Drawing for the job (mm, zero at the part's lowest x, y, z). Give positions to 0.01 mm unless a question says otherwise; leave off trailing zeros. Loops run counter-clockwise (first coordinate to the right, second up) from the corner with the lowest first, then second, coordinate; pieces in that order, holes last. Notation, with made-up numbers: M 45,66.5 L 88,66.5 A10 cw 88,76.5 Z; hole C 53.25,1.5 d4. An arc over 180 degrees is marked long. Use CSV: the item, a comma, the result in double quotes. Start each with the question number.
(1) Slice it at A-A on y = 7.5. List the corners of the cut face in (x, z), and give its area (3 significant figures).
(2) Slice it at C-C on x = 10. List the corners of the cut face in (y, z).
(3) Slice it at B-B on z = 13. List the corners of the cut face in (x, y), and give its area (3 significant figures).
(4) Wall check: line 1 along X through (y, z) = (8, 56.5); line 2 along X through (y, z) = (3.5, 51); line 3 along Z through (x, y) = (14, 0.5). Give the ranges that are in metal, low to high. Write a range as from..to.
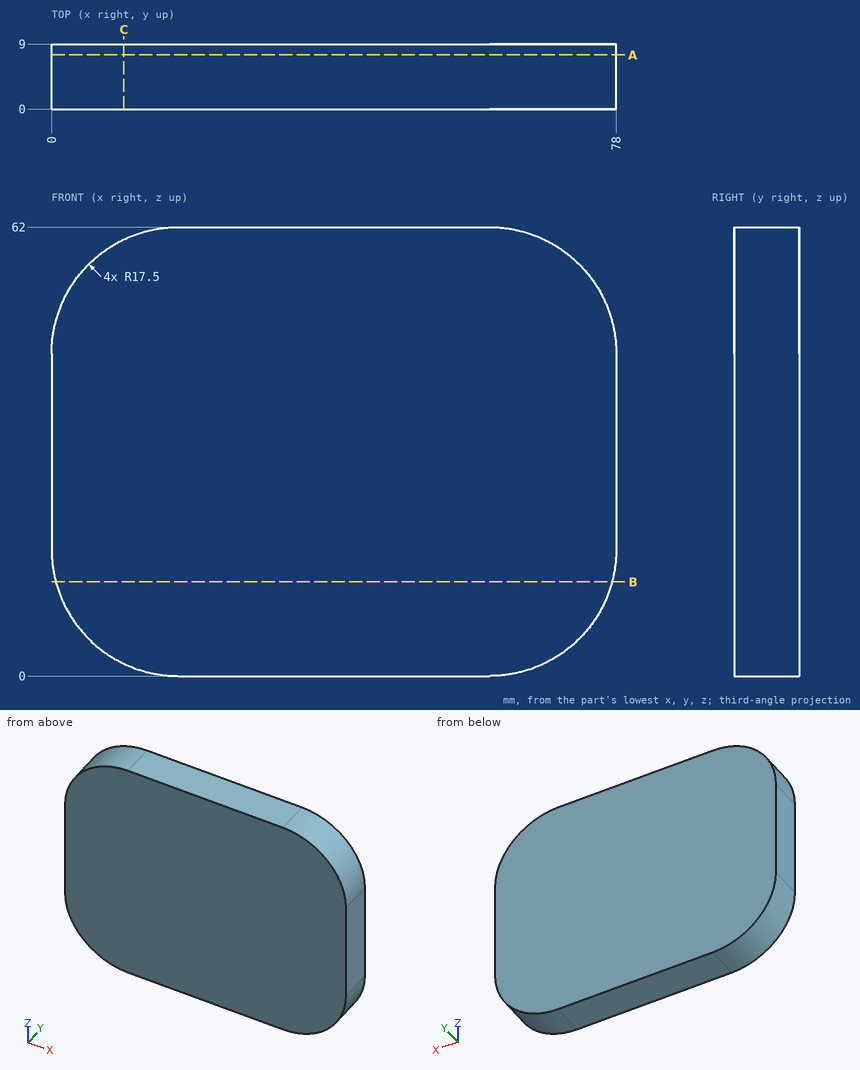
Reply:
1,outline,"M 0,17.5 A17.5 ccw 17.5,0 L 60.5,0 A17.5 ccw 78,17.5 L 78,44.5 A17.5 ccw 60.5,62 L 17.5,62 A17.5 ccw 0,44.5 Z"
1,area,"4,570 mm^2"
2,outline,"M 0,1.69 L 9,1.69 L 9,60.31 L 0,60.31 Z"
3,outline,"M 0.59,0 L 77.41,0 L 77.41,9 L 0.59,9 Z"
3,area,"691 mm^2"
4,line 1,"x = 4.76..73.24"
4,line 2,"x = 1.25..76.75"
4,line 3,"z = 0.35..61.65"
